from build123d import *

# Parameters (mm, degrees)
SKETCH_1_R          = 6
EXTRUDE_1_DEPTH     = 1
EXTRUDE_2_DEPTH     = 9
SKETCH_8_W          = 30
SKETCH_8_H          = 30
CUT_EXTRUDE_2_DEPTH = 4
SKETCH_9_R          = 6
EXTRUDE_6_DEPTH     = 4
SKETCH_10_R         = 5
EXTRUDE_7_DEPTH     = 6
SKETCH_11_R         = 11
CUT_EXTRUDE_3_DEPTH = 7
SKETCH_12_R         = 10
CUT_EXTRUDE_4_DEPTH = 10


with BuildPart() as part:
    # 스케치1 → 보스-돌출1 (new body)
    with BuildSketch(Plane(origin=(0, 0, 0), x_dir=(1, 0, 0), z_dir=(0, 1, 0))):
        Circle(SKETCH_1_R)
    extrude(amount=EXTRUDE_1_DEPTH)

    # 스케치2 → 보스-돌출2 (add)
    with BuildSketch(Plane(origin=(0, 1, 0), x_dir=(1, 0, 0), z_dir=(0, 1, 0))):
        with BuildLine():
            Line((-15, 0), (-15, -250))
            ThreePointArc((-15, -250), (0, -265), (15, -250))
            Line((15, -250), (15, 0))
            ThreePointArc((15, 0), (0, 15), (-15, 0))
        make_face()
    extrude(amount=EXTRUDE_2_DEPTH)

    # 스케치8 → 컷-돌출2 (cut)
    with BuildSketch(Plane(origin=(0, 10, 0), x_dir=(1, 0, 0), z_dir=(0, 1, 0))):
        with Locations((0, -250)):
            Rectangle(SKETCH_8_W, SKETCH_8_H)
    extrude(amount=-CUT_EXTRUDE_2_DEPTH, mode=Mode.SUBTRACT)

    # 스케치9 → 보스-돌출6 (add)
    with BuildSketch(Plane(origin=(0, 6, 0), x_dir=(1, 0, 0), z_dir=(0, 1, 0))):
        with Locations((0, -250)):
            Circle(SKETCH_9_R)
    extrude(amount=EXTRUDE_6_DEPTH)

    # 스케치10 → 보스-돌출7 (add)
    with BuildSketch(Plane(origin=(0, 10, 0), x_dir=(1, 0, 0), z_dir=(0, 1, 0))):
        with Locations((0, -250)):
            Circle(SKETCH_10_R)
    extrude(amount=EXTRUDE_7_DEPTH)

    # 스케치11 → 컷-돌출3 (cut)
    with BuildSketch(Plane.XZ):
        Circle(SKETCH_11_R)
    extrude(amount=-CUT_EXTRUDE_3_DEPTH, mode=Mode.SUBTRACT)

    # 스케치12 → 컷-돌출4 (cut, through all)
    with BuildSketch(Plane.XZ.offset(-7)):
        Circle(SKETCH_12_R)
    extrude(amount=-CUT_EXTRUDE_4_DEPTH, mode=Mode.SUBTRACT)


solid = part.part
Can you work these out from the model? Positions are in its coordinate system, mm. A direction names the side the tool comes from. Coordinates: 2 decimals unless noted, no trailing zeros. Write each loop counter-clockwise with the first axis right and the second up, starting at its lowest first coordinate (ties: lowest second). Pieces come first, ordered by that corner, then holes.
Q1. Imagine slicing it at C-C, the plane z = 93.5. List the corners of the cut face in (x, y) for me.
Results found:
outline: (-15, 1) - (15, 1) - (15, 10) - (-15, 10) - close
Q2. Which directions (+Z, -Z, +X, -X, +Y, -Y) give clear straight access to the entire face, cutting with the end or side of a thin tool? Please do faces 5 (the face through (0, 10, 108)), 6 (the face through (-4, 10, 246)), 7 (the face through (15, 5, 127)), 8 (the face through (2, 7, -10)), 9 (the face through (0, 3, 265)).
Results found:
face 5: -Z, +X, -X, +Y
face 6: +Y
face 7: +Z, -Z, +X, +Y, -Y
face 8: -Y
face 9: +Z, +Y, -Y
Q3. Imagine slicing it at B-B, the plane z = 7. List the corners of the cut face in (x, y) for me.
Results found:
outline: (-15, 1) - (-8.49, 1) - (-8.49, 7) - (-7.14, 7) - (-7.14, 10) - (-15, 10) - close; (7.14, 7) - (8.49, 7) - (8.49, 1) - (15, 1) - (15, 10) - (7.14, 10) - close
Q4. If we mould it in two halves opening along Z, with no side actions, what happens to faces 1 (the face through (-2.17, 8.48, -9.76)), 2 (the face through (0, 5, -15)), 3 (the face through (-2.38, 3.96, -10.74)), 4 (the face through (-15, 5, 123))? For each: +Z half, -Z half, draft (parallel to the pull), parting line (faces both ways), or undercut.
Results found:
face 1: undercut
face 2: -Z half
face 3: undercut
face 4: draft
Q5. Imagine slicing it at A-A, the plane x = 0. List the corners of the cut face in (y, z) for me, plus the area to 3 significant figures.
Results found:
outline: (1, -15) - (10, -15) - (10, -10) - (7, -10) - (7, -11) - (1, -11) - close; (1, 11) - (7, 11) - (7, 10) - (10, 10) - (10, 235) - (6, 235) - (6, 244) - (10, 244) - (10, 245) - (16, 245) - (16, 255) - (10, 255) - (10, 256) - (6, 256) - (6, 265) - (1, 265) - close
area: 2,320 mm2
Q6. For P1, Ø4, axis at x = -4, z = 60, coming from the +Y side; P2, Ø6, axis at x = 6.5, y = 9, coming from the -Z side; P3, Ø2, axis at x = -0.5, y = 8.5, coming from the +Z side, each with a flat end and sliding along its axis, tell me the tip position at first contact or that it passes through.
Results found:
P1: stops at y = 10
P2: stops at z = -14.59
P3: stops at z = 256
Q7. Please list where these lines run through material, in increasing order: L1, parallel to Z at x = 0, y = 7.65; L2, parallel to Z at x = 0, y = 2.9; L3, parallel to Y at x = 13, z = 77.
Results found:
L1: z = -15 to -10, 10 to 235, 244 to 256
L2: z = -15 to -11, 11 to 265
L3: y = 1 to 10
